Part model, mm, in its own coordinate system. A direction names the side the tool comes from. Round coordinates to 2 decimals unless told otherwise and drop trailing zeros. Write each loop counter-clockwise with the first axis right and the second up, starting at its lowest first coordinate (ties: lowest second). Pieces come first, ordered by that corner, then holes.
```python
from build123d import *
from build123d import SkipClean  # not in build123d's __all__

# Parameters (mm, degrees)
F1_R           = 8.89
F1_R_2         = 5.969
F3_R           = 7.62
F3_R_2         = 5.969
F4_R           = 7.62
F4_R_2         = 5.969
F5_DEPTH       = 5.08
F6_DEPTH       = 25.4
F6_DEPTH_BACK  = 25.4
F7_R           = 7.62
F8_R           = 7.62
F9_DEPTH       = 17.78
F0_W           = 25.4
F0_H           = 12.7
F10_DEPTH      = 8.89
F10_DEPTH_BACK = 8.89
F11_DEPTH      = 17.78


# Not quite as in the source:
# - a feature of the source that left no trace in its solid (it failed there, or was rolled back) is left out


with BuildPart() as f2:
    # F2: sweep along a path in F0
    with BuildLine(Plane.XY) as f2_path:
        Line((0, 0), (0, 35.9156))
        ThreePointArc((0, 35.9156), (12.7, 48.6156), (25.4, 35.9156))
        Line((25.4, 35.9156), (25.4, 0))
    # F1 (on Front) → F2 (sweep)
    with BuildSketch(Plane.XZ):
        Circle(F1_R)
        Circle(F1_R_2, mode=Mode.SUBTRACT)
    sweep(path=f2_path.line)

    # F3 (on face) + F4 (on face) → F5 (join)
    with BuildSketch(Plane.XZ):
        Circle(F3_R)
        Circle(F3_R_2, mode=Mode.SUBTRACT)
    with BuildSketch(Plane.XZ):
        with Locations((25.4, 0)):
            Circle(F4_R)
        with Locations((25.4, 0)):
            Circle(F4_R_2, mode=Mode.SUBTRACT)
    with SkipClean():  # cleaning this boolean's faces spoils the solid; the shape is the same uncleaned
        extrude(amount=F5_DEPTH)

    # F0 (on Top) → F6 (cut, two sides)
    with BuildSketch(Plane.XY) as f6_sk:
        with BuildLine():
            Line((-12.2957220301, 20.301265642), (0, 20.301265642))
            Line((0, 20.301265642), (0, 35.9156))
            ThreePointArc((0, 35.9156), (3.7197438789, 44.8958561211), (12.7, 48.6156))
            ThreePointArc((12.7, 48.6156), (21.6802561211, 44.8958561211), (25.4, 35.9156))
            Line((25.4, 35.9156), (25.4, 20.301265642))
            Line((25.4, 20.301265642), (40.2239970863, 20.301265642))
            Line((40.2239970863, 20.301265642), (40.2239970863, 60.9702691436))
            Line((40.2239970863, 60.9702691436), (-12.2957220301, 60.9702691436))
            Line((-12.2957220301, 60.9702691436), (-12.2957220301, 20.301265642))
        make_face()
        with BuildLine():
            Line((0, 35.9156), (0, 20.301265642))
            Line((0, 20.301265642), (12.7, 20.301265642))
            Line((12.7, 20.301265642), (12.7, 48.6156))
            ThreePointArc((12.7, 48.6156), (3.7197438789, 44.8958561211), (0, 35.9156))
        make_face()
        with BuildLine():
            Line((12.7, 20.301265642), (25.4, 20.301265642))
            Line((25.4, 20.301265642), (25.4, 35.9156))
            ThreePointArc((25.4, 35.9156), (21.6802561211, 44.8958561211), (12.7, 48.6156))
            Line((12.7, 48.6156), (12.7, 20.301265642))
        make_face()
    extrude(amount=-F6_DEPTH, mode=Mode.SUBTRACT)
    extrude(f6_sk.sketch, amount=F6_DEPTH_BACK, mode=Mode.SUBTRACT)

    # F7 (on face) + F8 (on face) → F9 (cut)
    with BuildSketch(Plane(origin=(0, 20.301265642, 0), x_dir=(-1, 0, 0), z_dir=(0, 1, 0))):
        with Locations((-25.4, 0)):
            Circle(F7_R)
    with BuildSketch(Plane(origin=(0, 20.301265642, 0), x_dir=(-1, 0, 0), z_dir=(0, 1, 0))):
        Circle(F8_R)
    extrude(amount=-F9_DEPTH, mode=Mode.SUBTRACT)

    # F0 (on Top) → F10 (join, two sides)
    with BuildSketch(Plane.XY) as f10_sk:
        with Locations((12.7, 11.9974283338)):
            Rectangle(F0_W, F0_H)
    extrude(amount=F10_DEPTH)
    extrude(f10_sk.sketch, amount=-F10_DEPTH_BACK)

    # F7 (on face) + F8 (on face) → F11 (cut)
    with BuildSketch(Plane(origin=(0, 20.301265642, 0), x_dir=(-1, 0, 0), z_dir=(0, 1, 0))):
        with Locations((-25.4, 0)):
            Circle(F7_R)
    with BuildSketch(Plane(origin=(0, 20.301265642, 0), x_dir=(-1, 0, 0), z_dir=(0, 1, 0))):
        Circle(F8_R)
    extrude(amount=-F11_DEPTH, mode=Mode.SUBTRACT)


solid = f2.part
```
Q1. Cut at C-C on z = -6.75. Write the cut outline in (x, y), plus the area to 3 significant figures.
Values follow:
outline: (-5.79, 0) - (-3.54, 0) - (-3.54, -5.08) - (3.54, -5.08) - (3.54, 0) - (5.79, 0) - (5.79, 5.65) - (19.61, 5.65) - (19.61, 0) - (21.86, 0) - (21.86, -5.08) - (28.94, -5.08) - (28.94, 0) - (31.19, 0) - (31.19, 20.3) - (28.94, 20.3) - (28.94, 2.52) - (21.86, 2.52) - (21.86, 20.3) - (19.61, 20.3) - (19.61, 18.35) - (5.79, 18.35) - (5.79, 20.3) - (3.54, 20.3) - (3.54, 2.52) - (-3.54, 2.52) - (-3.54, 20.3) - (-5.79, 20.3) - close
area: 466 mm2
Q2. Cut at A-A on x = -1. Write the cut outline in (y, z).
Values follow:
outline: (-5.08, -7.55) - (0, -7.55) - (0, -8.83) - (20.3, -8.83) - (20.3, -7.55) - (2.52, -7.55) - (2.52, -5.88) - (-5.08, -5.88) - close; (-5.08, 5.88) - (2.52, 5.88) - (2.52, 7.55) - (20.3, 7.55) - (20.3, 8.83) - (0, 8.83) - (0, 7.55) - (-5.08, 7.55) - close
Q3. Which spindle directions (+Z, -Z, +X, -X, +Y, -Y) get a long thin tool onto all of the face, cutting with end or side? Do faces 3 (the flat face through (13, 12, -8.89)), 4 (the cylindrical face through (1.65, 11.54, -7.44)), 5 (the cylindrical face through (-1.65, -2.5, -7.44)). Say none if no direction does.
Values follow:
face 3: -Z, +X, -X, +Y, -Y
face 4: +Y
face 5: -Y
Q4. Drop flat-ended pins along their axis: pin 1 (4 mm diameter, centred on y = 4, z = -5, fed in from -X); pin 2 (9 mm diameter, centred on x = 0, z = 0, fed in from -Y); pin 3 (2 mm diameter, centred on y = 4, z = 5, fed in from +X); pin 4 (8 mm diameter, centred on y = 13, z = 5.5, fed in from +X). Give the stop position or say it passes through.
Values follow:
pin 1: stops at x = -8.37
pin 2: passes through
pin 3: stops at x = 33.34
pin 4: stops at x = 34.16
Q5. Wall check: L1, parallel to X at y = 1.6, z = 0; L2, parallel to X at y = 7.25, z = 0.25; L3, parallel to X at y = -2, z = -4. Give the ranges that are in metal, low to high.
Values follow:
L1: x = -8.89 to -5.97, 5.97 to 8.89, 16.51 to 19.43, 31.37 to 34.29
L2: x = -8.89 to -7.62, 7.62 to 17.78, 33.02 to 34.29
L3: x = -6.49 to -4.43, 4.43 to 6.49, 18.91 to 20.97, 29.83 to 31.89
Q6. Cut at D-D on x = 26.5. Write the cut outline in (y, z), plus the area to 3 significant figures.
Values follow:
outline: (-5.08, -7.54) - (0, -7.54) - (0, -8.82) - (20.3, -8.82) - (20.3, -7.54) - (2.52, -7.54) - (2.52, -5.87) - (-5.08, -5.87) - close; (-5.08, 5.87) - (2.52, 5.87) - (2.52, 7.54) - (20.3, 7.54) - (20.3, 8.82) - (0, 8.82) - (0, 7.54) - (-5.08, 7.54) - close
area: 77.5 mm2
Q7. Cut at B-B on y = 10.5. Write the cut outline in (x, z), plus the area to 3 significant figures.
Values follow:
outline: (0, -8.89) - (25.4, -8.89) arc R8.89 ccw to (25.4, 8.89) - (0, 8.89) arc R8.89 ccw to start; hole circle Ø15.24 at (0, 0); hole circle Ø15.24 at (25.4, 0)
area: 335 mm2
Q8. Mould opens along X. For faces 1 (the cylindrical face through (17.787, -2.504, 0.335)), 2 (the flat face through (13, 12, 8.89)) say: +X half, -X half, draft (parallel to the pull), parting line (faces both ways), or undercut.
Values follow:
face 1: undercut
face 2: draft
